The model under review builds one solid part; all positions refer to its coordinate system, in mm. A direction names the side the tool comes from. Give positions to 0.01 mm unless a question says otherwise; leave off trailing zeros. Loops run counter-clockwise (first coordinate to the right, second up) from the corner with the lowest first, then second, coordinate; pieces in that order, holes last. Notation, with made-up numbers: M 89.5,54 L 118.5,54 A32 ccw 118.5,84 Z; hole C -11.75,-10.5 d11. An arc over 180 degrees is marked long. Put each result on its own line as item: value. Start each with the question number.
from build123d import *

# Parameters (mm, degrees)
F1_DEPTH = 13
F2_R     = 3
F3_DEPTH = 19.0259843945
F5_R     = 5.25
F6_DEPTH = 19
F9_D     = 3.3
F9_DEPTH = 8.1
F9_START = 1.0431091
F9_TIP   = 0.9914200214


with BuildPart() as f1:
    # F0 (on Front) → F1 (new body)
    with BuildSketch(Plane.XZ):
        with BuildLine():
            ThreePointArc((1, 8.94427191), (9, 0), (1, -8.94427191))
            Line((1, -8.94427191), (1, -20))
            ThreePointArc((1, -20), (20.0249843945, 0), (1, 20))
            Line((1, 20), (1, 8.94427191))
        make_face()
    extrude(amount=F1_DEPTH)

    # F2 (on face) → F3 (cut, through all)
    with BuildSketch(Plane(origin=(1, 0, 0), x_dir=(0, -1, 0), z_dir=(-1, 0, 0))):
        with Locations((6.5, 13.5)):
            Circle(F2_R)
        with Locations((6.5, -13.5)):
            Circle(F2_R)
    extrude(amount=-F3_DEPTH, mode=Mode.SUBTRACT)

    # F5 (on offset) → F6 (cut)
    with BuildSketch(Plane(origin=(26, 0, 0), x_dir=(0, -1, 0), z_dir=(-1, 0, 0))):
        with Locations((6.5, -13.5)):
            Circle(F5_R)
        with Locations((6.5, 13.5)):
            Circle(F5_R)
    extrude(amount=F6_DEPTH, mode=Mode.SUBTRACT)

    # F9
    # its depths count from where the whole tool has entered the part; down to there all is cleared
    with Locations(Plane(origin=(21, 0, 0), x_dir=(0, -1, 0), z_dir=(1, 0, 0)).offset(-F9_START)):
        with Locations((6.5, 0)):
            Hole(F9_D / 2, depth=F9_DEPTH)
            with Locations((0, 0, -(F9_DEPTH + F9_TIP / 2))):  # 118° drill point
                Cone(0, F9_D / 2, F9_TIP, mode=Mode.SUBTRACT)


solid = f1.part
(1) For faces 1 (the cylindrical face through (15.88, -8.15, -0.07)), 2 (the cylindrical face through (20.02, -3.52, -0.43)), list the 3-axis set-ups (+Z, -Z, +X, -X, +Y, -Y) from which the entire face can be reached by the end or side of a thin tool; tool diameter is ignored.
(2) We need section B-B, the plane z = -13.5. Write out the cut boundary in (x, y), plus the area to 3 significant figures.
(3) We need section A-A, the plane x = 4. Write out the cut boundary in (y, z).
(4) We need section D-D, the plane y = -6. State how many separate pieces and enclosed holes the cut face has, plus the area to 3 significant figures.
(5) To check wall thickness, follow L1, parallel to Y at x = 10.25, z = -13.5; L2, parallel to Z at x = 5.1, y = -6.5; L3, parallel to Z at x = 5.65, y = -6.5. State the ranges of each line that lie inside material, in increasing order. Write a range as [from, to].
(6) Insertion check: pin 1 (10 mm diameter, centred on x = 9.5, z = 10.5, fed in from +Y); pin 2 (6 mm diameter, centred on x = 17, y = -4.5, fed in from +Z); pin 3 (6 mm diameter, centred on x = 11, y = -2.5, fed in from +Z); pin 4 (6 mm diameter, centred on y = -2.5, z = -11.5, fed in from +X). Each pin has a flat end and moves straight along its axis. Give the tip position at first contact, or say it passes through.
(7) Draft analysis for pull direction Y (two halves, no side actions). For faces 3 (the flat face through (10, -13, 0)), 4 (the cylindrical face through (9, -6, 0)), 5 (the cylindrical face through (11.452, -5.817, -8.295)), state which applies: +Y half, -Y half, draft (parallel to the pull), parting line (faces both ways), or undercut.
Check sheet entries:
1. face 1: +X
1. face 2: +X, +Y, -Y
2. outline: M 1,-13 L 14.79,-13 L 14.79,-11.75 L 7,-11.75 L 7,-9.5 L 1,-9.5 Z; M 1,-3.5 L 7,-3.5 L 7,-1.25 L 14.79,-1.25 L 14.79,0 L 1,0 Z
2. area: 61.5 mm²
3. outline: M -13,-19.62 L 0,-19.62 L 0,-8.06 L -13,-8.06 Z; M -13,8.06 L 0,8.06 L 0,19.62 L -13,19.62 Z; hole C -6.5,-13.5 d6; hole C -6.5,13.5 d6
4. separate pieces: 3
4. enclosed holes: 0
4. area: 233 mm²
5. L1: y = [-13, -11.75], [-1.25, 0]
5. L2: z = [-19.36, -16.5], [-10.5, -7.42], [7.42, 10.5], [16.5, 19.36]
5. L3: z = [-19.21, -16.5], [-10.5, -7.01], [7.01, 10.5], [16.5, 19.21]
6. pin 1: stops at y = 0
6. pin 2: stops at z = 11.65
6. pin 3: stops at z = 18.36
6. pin 4: stops at x = 18.13
7. face 3: -Y half
7. face 4: draft
7. face 5: undercut
